Geometry: final body of the model. Coordinates: model frame, mm. Face numbers are marked on the shaded views. A direction names the side the tool comes from. Give positions to 0.01 mm unless a question says otherwise; leave off trailing zeros. Loops run counter-clockwise (first coordinate to the right, second up) from the corner with the lowest first, then second, coordinate; pieces in that order, holes last. Notation, with made-up numbers: (39, 53) -> (75, 53) arc R23 cw to (75, 79) -> close; hole circle Ø3 at (74.25, 47). An arc over 180 degrees is marked (long way). Answer in a Markdown table with one row per item. Add a question column.
1) Section query C-C (z = 33). Return the cut outline in (x, y), plus the area to 3 significant figures.
2) First-contact query: P1, Ø12, axis at y = 193.5, z = 54.5, coming from the -X side; P2, Ø2, axis at y = 115.5, z = 98, coming from the +X side; P3, Ø8, axis at x = -72, z = 52, coming from the -Y side. Flat tips, straight axial feed; report the tip coordinate or a pass-through.
3) Access query for the marked faces 1, 2 and 3. Directions: +Z, -Z, +X, -X, +Y, -Y. A direction counts if a zero-diameter tool reaches every point of the face in a straight line with its end or side. Return the directions, or none.
4) Line query: line 1 (Y direction, x = 12, z = 60); line 2 (Z direction, x = 20, y = 214.25); line 3 (X direction, y = 217.75, z = 60). Output: solid intervals per line, ascending. Write a range as from..to.
5) Section query B-B (x = 120). Return the cut outline in (y, z), plus the area to 3 significant figures.
6) Section query A-A (y = 58.25). Return the cut outline in (x, z).
7) Section query D-D (x = 90). Return the cut outline in (y, z), plus the area to 3 significant figures.
```python
from build123d import *

# Parameters (mm, degrees)
EXTRUDE_1_DEPTH          = 120
SKETCH_2_R               = 4
SKETCH_2_R_2             = 2.139034835
CUT_EXTRUDE_1_DEPTH      = 100
SKETCH_3_R               = 4
CUT_EXTRUDE_2_DEPTH      = 1
CUT_EXTRUDE_2_DEPTH_BACK = 10


with BuildPart() as part:
    # 草图1 → 凸台-拉伸1 (new body)
    with BuildSketch(Plane.XY):
        Polygon((0, 0), (40, 0), (40, 210), (140, 210), (140, 220), (-100, 220), (-100, 210), (0, 210), align=None)
    extrude(amount=EXTRUDE_1_DEPTH)

    # 草图2 → 切除-拉伸1 (cut)
    with BuildSketch(Plane(origin=(40, 0, 0), x_dir=(0, 0, -1), z_dir=(1, 0, 0))):
        with Locations((-60, 58.25)):
            Circle(SKETCH_2_R)
        with Locations((-60, 100.75)):
            Circle(SKETCH_2_R_2)
        with Locations((-23.193920339, 79.5)):
            Circle(SKETCH_2_R_2)
        with Locations((-23.193920339, 37)):
            Circle(SKETCH_2_R_2)
        with Locations((-60, 15.75)):
            Circle(SKETCH_2_R_2)
        with Locations((-96.806079661, 37)):
            Circle(SKETCH_2_R_2)
        with Locations((-96.806079661, 79.5)):
            Circle(SKETCH_2_R_2)
    extrude(amount=-CUT_EXTRUDE_1_DEPTH, mode=Mode.SUBTRACT)

    # 草图3 → 切除-拉伸2 (cut, two sides)
    with BuildSketch(Plane(origin=(0, 220, 0), x_dir=(1, 0, 0), z_dir=(0, 1, 0))) as cut_extrude_2_sk:
        with Locations((-80, -60)):
            Circle(SKETCH_3_R)
        with Locations((20, -20)):
            Circle(SKETCH_3_R)
        with Locations((120, -60)):
            Circle(SKETCH_3_R)
        with Locations((20, -100)):
            Circle(SKETCH_3_R)
    extrude(amount=CUT_EXTRUDE_2_DEPTH, mode=Mode.SUBTRACT)
    extrude(cut_extrude_2_sk.sketch, amount=-CUT_EXTRUDE_2_DEPTH_BACK, mode=Mode.SUBTRACT)


solid = part.part
```
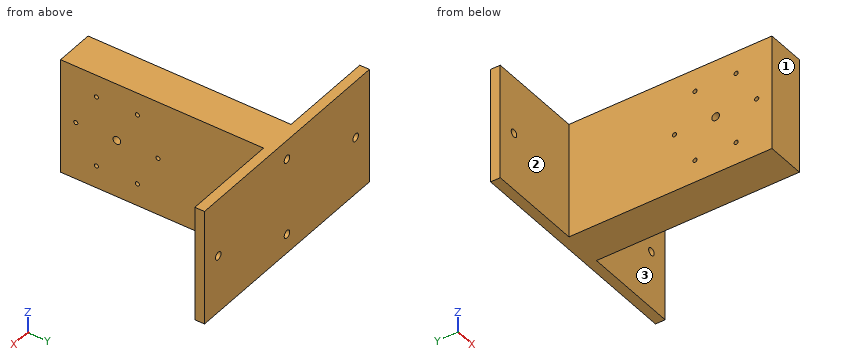
Evaluation:
| question | item | result |
|---|---|---|
| 1 | outline | (-100, 210) -> (0, 210) -> (0, 0) -> (40, 0) -> (40, 210) -> (140, 210) -> (140, 220) -> (-100, 220) -> close |
| 1 | area | 10,800 mm² |
| 2 | P1 | x = 0 |
| 2 | P2 | x = 40 |
| 2 | P3 | y = 210 |
| 3 | face 1 | +Z, -Z, +X, -X, -Y |
| 3 | face 2 | +Z, -Z, -X, -Y |
| 3 | face 3 | +Z, -Z, +X, -Y |
| 4 | line 1 | 0..13.61, 17.89..54.25, 62.25..98.61, 102.89..220 |
| 4 | line 2 | 0..16, 24..96, 104..120 |
| 4 | line 3 | -100..-84, -76..116, 124..140 |
| 5 | outline | (210, 0) -> (220, 0) -> (220, 56) -> (210, 56) -> close; (210, 64) -> (220, 64) -> (220, 120) -> (210, 120) -> close |
| 5 | area | 1,120 mm² |
| 6 | outline | (0, 0) -> (40, 0) -> (40, 56) -> (0, 56) -> close; (0, 64) -> (40, 64) -> (40, 120) -> (0, 120) -> close |
| 7 | outline | (210, 0) -> (220, 0) -> (220, 120) -> (210, 120) -> close |
| 7 | area | 1,200 mm² |
